Geometry: final body of the model. Coordinates: model frame, mm. A direction names the side the tool comes from. Round coordinates to 2 decimals unless told otherwise and drop trailing zeros. Write each loop counter-clockwise with the first axis right and the second up, starting at its lowest first coordinate (ties: lowest second). Pieces come first, ordered by that corner, then holes. Notation, with made-up numbers: M 70,70.5 L 110,70.5 A22 ccw 110,94.5 Z; hole C -2.5,87.25 d11. An arc over 180 degrees is marked long. Use one line per item in the form item = value. Start each with the question number.
Item 1: Pull-direction query (X, two-part tool) for faces 3 (the flat face through (-3, 50, 758)), 4 (the cylindrical face through (214.98, 1.98, 478.21)), 5 (the cylindrical face through (34.608, -69.72, 926.538)); classes: pulls with the +X half, pulls with the -X half, needs draft (parallel to the pull), parting line crosses it, or undercut.
Item 2: Section query D-D (y = 0). Return loops of the section in (x, z), and give its area (3 significant figures).
Item 3: Reachability of faces 1 (the flat face through (3, 1, 0)), 2 (the flat face through (-3, -50, 758)) from +Z, -Z, +X, -X, +Y, -Y: full face, straight path, thin tool, end or side. Return the list, or none.
Item 4: Section query B-B (x = -36). Return loops of the section in (y, z).
Item 5: Pin query (flat end, axial travel): pin 1 Ø5 at (x, z) = (-155.5, 698.5) entering from +Y; pin 2 Ø5 at (y, z) = (13, 399) entering from -X; pin 3 Ø6 at (x, y) = (17.5, 7.5) entering from +Z. Return the tip coordinate at first contact, or that it passes through.
Item 6: Ray query, probe 1 along Z at (x, y) = (0, 63); probe 2 along Y at (x, z) = (-61.5, 639); probe 3 along Z at (x, y) = (0, -58). Return the intervals inside material, ascending.
Item 7: Section query C-C (x = -103.5). Return loops of the section in (y, z), and give its area (3 significant figures).
Item 8: Section query A-A (z = 860). Return loops of the section in (x, y), and give its area (3 significant figures).
from build123d import *

# Parameters (mm, degrees)
BOSS_EXTRUDE1_DEPTH = 1000
FILLET1_R           = 30
SKETCH2_W           = 431.388380784
SKETCH2_H           = 100
CUT_EXTRUDE1_DEPTH  = 400
SKETCH3_R           = 75
CUT_EXTRUDE2_DEPTH  = 181.0000001


with BuildPart() as part:
    # Sketch1 → Boss-Extrude1 (new body)
    with BuildSketch(Plane.XY):
        with BuildLine():
            Line((-125, 90), (125, 90))
            ThreePointArc((125, 90), (215, 0), (125, -90))
            Line((125, -90), (-125, -90))
            ThreePointArc((-125, -90), (-215, 0), (-125, 90))
        make_face()
    extrude(amount=BOSS_EXTRUDE1_DEPTH)

    # Fillet1
    fillet1_edges = [part.edges().sort_by_distance(p)[0] for p in [
        (215, 0, 1000),
        (0, 90, 1000),
        (-215, 0, 1000),
        (0, -90, 1000),
    ]]
    fillet(fillet1_edges, radius=FILLET1_R)

    # Sketch2 → Cut-Extrude1 (cut)
    with BuildSketch(Plane.XY.offset(1000)):
        with Locations((-0.091183766, 0)):
            Rectangle(SKETCH2_W, SKETCH2_H)
    extrude(amount=-CUT_EXTRUDE1_DEPTH, mode=Mode.SUBTRACT)

    # Sketch3 → Cut-Extrude2 (cut, through all)
    with BuildSketch(Plane(origin=(0, 90, 0), x_dir=(1, 0, 0), z_dir=(0, 1, 0))):
        with Locations((0, -860)):
            Circle(SKETCH3_R)
    extrude(amount=-CUT_EXTRUDE2_DEPTH, mode=Mode.SUBTRACT)


solid = part.part
Working result:
q1.face_3 = needs draft
q1.face_4 = pulls with the +X half
q1.face_5 = undercut
q2.outline = M -215,0 L 215,0 L 215,600 L -215,600 Z
q2.area = 258,000 mm²
q3.face_1 = -Z, +X, -X, +Y, -Y
q3.face_2 = +Z, +X, -X
q4.outline = M -90,0 L 90,0 L 90,794.2 L 50,794.2 L 50,600 L -50,600 L -50,794.2 L -90,794.2 Z; M -90,925.8 L -50,925.8 L -50,1000 L -60,1000 A30 ccw -90,970 Z; M 50,925.8 L 90,925.8 L 90,970 A30 ccw 60,1000 L 50,1000 Z
q5.pin_1 = 85.53
q5.pin_2 = -214.39
q5.pin_3 = 600
q6.probe_1 = 0 to 785, 935 to 999.85
q6.probe_2 = -90 to -50, 50 to 90
q6.probe_3 = 0 to 785, 935 to 1000
q7.outline = M -90,0 L 90,0 L 90,970 A30 ccw 60,1000 L 50,1000 L 50,600 L -50,600 L -50,1000 L -60,1000 A30 ccw -90,970 Z
q7.area = 140,000 mm²
q8.outline = M -199.83,-50 A90 ccw -125,-90 L -75,-90 L -75,-50 Z; M -199.83,50 L -75,50 L -75,90 L -125,90 A90 ccw Z; M 75,-90 L 125,-90 A90 ccw 199.83,-50 L 75,-50 Z; M 75,50 L 199.83,50 A90 ccw 125,90 L 75,90 Z
q8.area = 16,400 mm²
